from build123d import *

# Parameters (mm, degrees)
BOSS_EXTRUDE1_DEPTH = 30
FILLET1_R           = 3
FILLET2_R           = 0.5
FILLET3_R           = 1
SKETCH3_R           = 15
BOSS_EXTRUDE2_DEPTH = 5
SKETCH4_R           = 10.5
CUT_EXTRUDE2_DEPTH  = 7


with BuildPart() as part:
    # Sketch1 → Boss-Extrude1 (new body)
    with BuildSketch(Plane.XY):
        Polygon((0, 0), (0, 40), (12.5, 40), (12.5, 15), (10.5, 15), (10.5, 38), (6.7, 38), (4, 33.5), (4, 0), align=None)
    extrude(amount=BOSS_EXTRUDE1_DEPTH)

    # Fillet1
    fillet1_edges = [part.edges().sort_by_distance(p)[0] for p in [
        (0, 40, 15),
        (12.5, 40, 15),
    ]]
    fillet(fillet1_edges, radius=FILLET1_R)

    # Fillet2
    fillet2_edges = [part.edges().sort_by_distance(p)[0] for p in [
        (10.5, 38, 15),
    ]]
    fillet(fillet2_edges, radius=FILLET2_R)

    # Fillet3
    fillet3_edges = [part.edges().sort_by_distance(p)[0] for p in [
        (12.5, 15, 15),
    ]]
    fillet(fillet3_edges, radius=FILLET3_R)

    # Sketch3 → Boss-Extrude2 (add)
    with BuildSketch(Plane.ZY):
        with Locations((15, 18)):
            Circle(SKETCH3_R)
    extrude(amount=BOSS_EXTRUDE2_DEPTH)

    # Sketch4 → Cut-Extrude2 (cut)
    with BuildSketch(Plane.ZY.offset(5)):
        with Locations((15, 18)):
            Circle(SKETCH4_R)
    extrude(amount=-CUT_EXTRUDE2_DEPTH, mode=Mode.SUBTRACT)


solid = part.part
Work out the finished part from the listing and answer in its coordinate system (mm). A direction names the side the tool comes from. Round coordinates to 2 decimals unless told otherwise and drop trailing zeros. Write each loop counter-clockwise with the first axis right and the second up, starting at its lowest first coordinate (ties: lowest second). Pieces come first, ordered by that corner, then holes. Notation, with made-up numbers: (21, -6.75) - (33, -6.75) arc R13 cw to (33, 1.25) - close; hole circle Ø11 at (2, 54.25). An arc over 180 degrees is marked (long way). Answer in a Markdown table with one row per item. Add a question column.
1. A cutting plane is placed at D-D, the plane y = 13. Determine the outline of the cut face in (x, z).
2. The mould has two halves that part along Z. Classify faces 4 (the cylindrical face through (-1.549, 26.854, 20.645)), 5 (the flat face through (2, 0, 15)), 6 (the flat face through (3.6, 24.7, 0)), 7 (the cylindrical face through (-2.465, 3.357, 11.748)): +Z half, -Z half, draft (parallel to the pull), parting line (faces both ways), or undercut.
3. Find the intervals of material crossed by line 1 along Y through (x, z) = (-1.5, 15); line 2 along Y through (x, z) = (9.25, 2.5); line 3 along X through (y, z) = (19.5, 10.75), in increasing order. Write a range as from..to.
4. Given pin 1 (6.5 mm diameter, centred on y = 23, z = 11.5, fed in from -X); pin 2 (2.5 mm diameter, centred on x = 8.5, z = 8, fed in from -Y); pin 3 (2 mm diameter, centred on x = 7.5, z = 23.5, fed in from -Y), each flat-ended and moving along its own axis, determine where each tip first touches the part or whether it passes through.
5. For faces 1 (the flat face through (4, 17, 15)), 2 (the flat face through (0, 34, 15)), 3 (the flat face through (11, 15, 15)), determine the directions among +Z, -Z, +X, -X, +Y, -Y from which every point of the face is accessible in a straight line to the end or side of a thin tool.
6. A cutting plane is placed at C-C, the plane x = -0.75. Determine the outline of the cut face in (y, z).
7. A cutting plane is placed at A-A, the plane y = 31. Determine the outline of the cut face in (x, z).
8. A cutting plane is placed at B-B, the plane z = 15. Determine the outline of the cut face in (x, y).
Worked out:
| question | item | result |
|---|---|---|
| 1 | outline | (-5, 0.86) - (0, 0.86) - (0, 0) - (4, 0) - (4, 30) - (0, 30) - (0, 29.14) - (-5, 29.14) - (-5, 24.23) - (2, 24.23) - (2, 5.77) - (-5, 5.77) - close |
| 2 | face 4 | undercut |
| 2 | face 5 | draft |
| 2 | face 6 | -Z half |
| 2 | face 7 | parting line |
| 3 | line 1 | 3..7.5, 28.5..33 |
| 3 | line 2 | 38..40 |
| 3 | line 3 | 2..4, 10.5..12.5 |
| 4 | pin 1 | x = 2 |
| 4 | pin 2 | y = 38 |
| 4 | pin 3 | y = 37.67 |
| 5 | face 1 | +Z, -Z, -Y |
| 5 | face 2 | -X, +Y |
| 5 | face 3 | +Z, -Z, +X, -Y |
| 6 | outline | circle Ø30 at (18, 15); hole circle Ø21 at (18, 15) |
| 7 | outline | (-5, 7.52) - (0, 7.52) - (0, 0) - (4, 0) - (4, 30) - (0, 30) - (0, 22.48) - (-5, 22.48) - close; (10.5, 0) - (12.5, 0) - (12.5, 30) - (10.5, 30) - close |
| 8 | outline | (-5, 3) - (0, 3) - (0, 0) - (4, 0) - (4, 33.5) - (6.7, 38) - (10, 38) arc R0.5 cw to (10.5, 37.5) - (10.5, 15) - (11.5, 15) arc R1 ccw to (12.5, 16) - (12.5, 37) arc R3 ccw to (9.5, 40) - (3, 40) arc R3 ccw to (0, 37) - (0, 33) - (-5, 33) - (-5, 28.5) - (2, 28.5) - (2, 7.5) - (-5, 7.5) - close |
